Can you work these out from the model? Positions are in its coordinate system, mm. Face numbers are marked on the shaded views. Round coordinates to 2 decimals unless told otherwise and drop trailing zeros. Loops run counter-clockwise (first coordinate to the right, second up) from the corner with the lowest first, then second, coordinate; pieces in that order, holes last. Notation, with made-up numbers: M -2,70.5 L 28,70.5 A24 ccw 28,98.5 Z; hole C 0,89.5 d11. An arc over 180 degrees is marked long. Return JSON: item names as keys, results as strings.
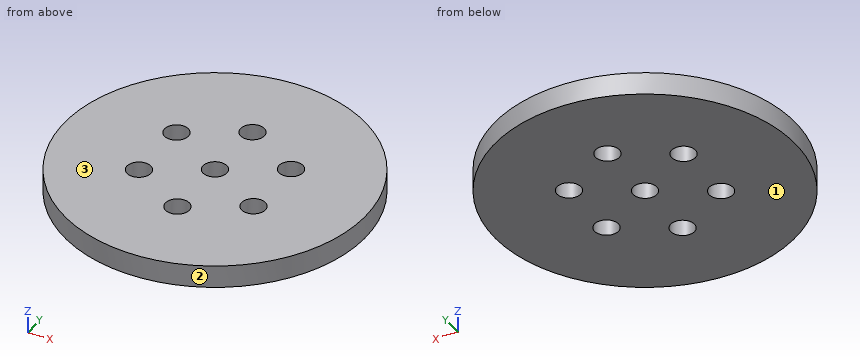
```python
from build123d import *

# Parameters (mm, degrees)
F0_R     = 20
F0_R_2   = 1.5875
F1_DEPTH = 3


with BuildPart() as f1:
    # F0 (on Top) → F1 (new body)
    with BuildSketch(Plane.XY):
        with Locations((-36.162619, 9.984028)):
            Circle(F0_R)
        with Locations((-43.817643, 5.564397)):
            Circle(F0_R_2, mode=Mode.SUBTRACT)
        with Locations((-36.162619, 1.144767)):
            Circle(F0_R_2, mode=Mode.SUBTRACT)
        with Locations((-28.507594, 5.564397)):
            Circle(F0_R_2, mode=Mode.SUBTRACT)
        with Locations((-43.817643, 14.403658)):
            Circle(F0_R_2, mode=Mode.SUBTRACT)
        with Locations((-36.162619, 9.984028)):
            Circle(F0_R_2, mode=Mode.SUBTRACT)
        with Locations((-28.507594, 14.403658)):
            Circle(F0_R_2, mode=Mode.SUBTRACT)
        with Locations((-36.162619, 18.823288)):
            Circle(F0_R_2, mode=Mode.SUBTRACT)
    extrude(amount=F1_DEPTH)


solid = f1.part
```
Q1. If I drill on line 1 along X through (y, z) = (14, 2.05); line 2 along Y through (x, z) = (-29, 0.95); line 3 along Y through (x, z) = (-35, 0.7), over which ranges is the centre line in solid material (lowest first)?
Results:
{"line 1": "x = -55.76 to -45.35, -42.28 to -30.04, -26.97 to -16.57", "line 2": "y = -8.69 to 4.06, 7.07 to 12.89, 15.91 to 28.66", "line 3": "y = -9.98 to 0.06, 2.23 to 8.9, 11.06 to 17.74, 19.9 to 29.95"}
Q2. Thinking about a two-plate mould opening in Z: for the marked faces 1, 2 and 3, which applies, pulls with the +Z half, pulls with the -Z half, needs draft (parallel to the pull), parting line crosses it, or undercut?
Results:
{"face 1": "pulls with the -Z half", "face 2": "needs draft", "face 3": "pulls with the +Z half"}
Q3. Suppose I cut it at A-A, the plane x = -27.5. Please give me the cut outline in (y, z).
Results:
{"outline": "M -8.04,0 L 4.34,0 L 4.34,3 L -8.04,3 Z; M 6.79,0 L 13.18,0 L 13.18,3 L 6.79,3 Z; M 15.63,0 L 28.01,0 L 28.01,3 L 15.63,3 Z"}
Q4. Suppose I cut it at B-B, the plane y = 15. Please give me the cut outline in (x, z).
Results:
{"outline": "M -55.52,0 L -45.29,0 L -45.29,3 L -55.52,3 Z; M -42.35,0 L -29.98,0 L -29.98,3 L -42.35,3 Z; M -27.04,0 L -16.8,0 L -16.8,3 L -27.04,3 Z"}
Q5. Suppose I cut it at D-D, the plane y = -3. Please give me the cut outline in (x, z).
Results:
{"outline": "M -51.37,0 L -20.95,0 L -20.95,3 L -51.37,3 Z"}
Q6. Suppose I cut it at C-C, the plane z = 0.65. Please give me the cut outline in (x, y) (1 decimal), plus the area to 3 significant figures.
Results:
{"outline": "C -36.2,10 d40; hole C -43.8,5.6 d3.2; hole C -43.8,14.4 d3.2; hole C -36.2,1.1 d3.2; hole C -36.2,10 d3.2; hole C -36.2,18.8 d3.2; hole C -28.5,5.6 d3.2; hole C -28.5,14.4 d3.2", "area": "1,200 mm2"}
